Part print with two shaded views. Sizes in mm from the minimum x, y, z corner. A direction names the side the tool comes from. Round coordinates to 2 decimals unless told otherwise and drop trailing zeros. Order: outer loops, then holes, each group sorted by start corner. A loop starts at its lowest first (then second) coordinate and runs counter-clockwise, first axis right, second up. Notation, with made-up numbers: (-39.75, -31) -> (-0.75, -31) arc R33 ccw to (-0.75, 2) -> close; hole circle Ø3 at (3.25, 16.5). An arc over 180 degrees is marked (long way). Put each result on its own line as item: value. Start each with the question number.
Q1. Probe L1, parallel to X at y = 27, z = 110.5; L2, parallel to Z at x = 36, y = 20; L3, parallel to Z at x = 26, y = 20. List the from-to ranges inside material, lowest first.
Q2. Cut at B-B, the plane z = 105. List the corners of the cut face in (x, y), and give its area (3 significant figures).
Q3. 3-axis set-ups, long thin cutter, end or side, ignore diameter. For the marked faces 5 and 6: which of +Z, -Z, +X, -X, +Y, -Y reach the whole face in a straight line?
Q4. Cut at D-D, the plane x = 33. List the corners of the cut face in (y, z), and give its area (3 significant figures).
Q5. Flat gauge pins, fed straight in: P1, Ø10, axis at x = 21.5, y = 26.5, coming from the +Z side; P2, Ø4, axis at x = 20, y = 20, coming from the -Z side; P3, Ø8, axis at x = 23, z = 108, coming from the -Y side. Where does each tip first touch, or does it go through?
Q6. Cut at A-A, the plane y = 20. List the corners of the cut face in (x, z), and give its area (3 significant figures).
Q7. Cut at C-C, the plane y = 8. List the corners of the cut face in (x, z), and give its area (3 significant figures).
Q8. Pull direction X, two halves, no side cores. Call the marked faces 1, 2, 3 and 4: released by +X, released by -X, zero draft, split by the parting line, or undercut.
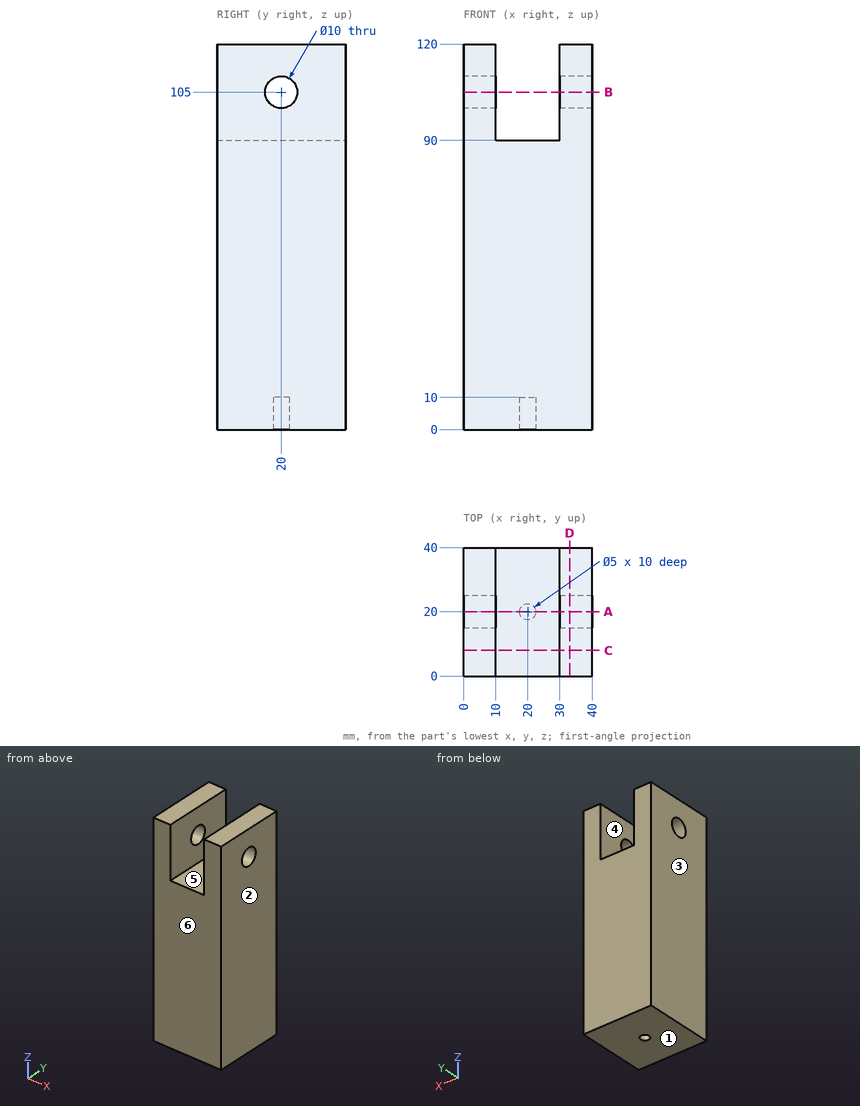
Ans:
1. L1: x = 0 to 10, 30 to 40
1. L2: z = 0 to 100, 110 to 120
1. L3: z = 0 to 90
2. outline: (0, 0) -> (10, 0) -> (10, 15) -> (0, 15) -> close; (0, 25) -> (10, 25) -> (10, 40) -> (0, 40) -> close; (30, 0) -> (40, 0) -> (40, 15) -> (30, 15) -> close; (30, 25) -> (40, 25) -> (40, 40) -> (30, 40) -> close
2. area: 600 mm^2
3. face 5: +Z, +Y, -Y
3. face 6: +Z, -Z, +X, -X, -Y
4. outline: (0, 0) -> (40, 0) -> (40, 120) -> (0, 120) -> close; hole circle Ø10 at (20, 105)
4. area: 4,720 mm^2
5. P1: stops at z = 90
5. P2: stops at z = 10
5. P3: passes through
6. outline: (0, 0) -> (17.5, 0) -> (17.5, 10) -> (22.5, 10) -> (22.5, 0) -> (40, 0) -> (40, 100) -> (30, 100) -> (30, 90) -> (10, 90) -> (10, 100) -> (0, 100) -> close; (0, 110) -> (10, 110) -> (10, 120) -> (0, 120) -> close; (30, 110) -> (40, 110) -> (40, 120) -> (30, 120) -> close
6. area: 3,950 mm^2
7. outline: (0, 0) -> (40, 0) -> (40, 120) -> (30, 120) -> (30, 90) -> (10, 90) -> (10, 120) -> (0, 120) -> close
7. area: 4,200 mm^2
8. face 1: zero draft
8. face 2: released by +X
8. face 3: released by -X
8. face 4: undercut
